Here's how the part is built. I have some questions about the finished solid (model axes, mm). Coordinates: 2 decimals unless noted, no trailing zeros. Write each loop counter-clockwise with the first axis right and the second up, starting at its lowest first coordinate (ties: lowest second). Pieces come first, ordered by that corner, then holes.
Autodesk Inventor part; units mm, degrees
ref_plane "YZ Plane" through (0, 0, 0) normal (1, 0, 0) x (0, 1, 0)
ref_plane "XZ Plane" through (0, 0, 0) normal (0, 1, 0) x (-1, 0, 0)
ref_plane "XY Plane" through (0, 0, 0) normal (0, 0, 1) x (1, 0, 0)
sketch "Sketch1" plane through (0, 0, 0) normal (0, 1, 0) x (-1, 0, 0)
  line L0 (0, 0) -> (1000, 0)
  line L1 (1000, 0) -> (1000, 1500)
  line L2 (1000, 1500) -> (0, 1500)
  line L3 (0, 1500) -> (0, 0)
  dimension "d0" = 1000
  dimension "d1" = 1500
extrude "base" add sketch "Sketch1" along normal blind 150
sketch "Sketch2" plane through (0, 150, 0) normal (0, 1, 0) x (1, 0, 0)
  circle A0 centre (-500, -700) radius 57.5
  line L0 (0, 0) -> (-1000, 0)
  line L1 (-1000, -1500) -> (0, -1500)
  line L2 (-500, 0) -> (-500, -1500) construction
  dimension "d4" = 115
  dimension "d38" = 700
extrude "air" cut sketch "Sketch2" against normal through all
sketch "Sketch3" plane through (0, 150, 0) normal (0, 1, 0) x (1, 0, 0)
  circle A0 centre (-500, -700) radius 57.5
  circle A1 centre (-400, -200) radius 24.5
  circle A2 centre (-600, -200) radius 24.5
  line L0 (0, 0) -> (-1000, 0)
  dimension "d7" = 49
  dimension "d40" = 100
  dimension "d41" = 49
  dimension "d42" = 100
  dimension "d55" = 200
extrude "power" cut sketch "Sketch3" against normal blind 254 contours A1 | A2
sketch "Sketch4" plane through (0, 150, 0) normal (0, 1, 0) x (1, 0, 0)
  circle A0 centre (-600, -200) radius 24.5
  circle A1 centre (-500, -500) radius 24.5
  line L0 (0, 0) -> (-1000, 0)
  dimension "d52" = 49
  dimension "d53" = 500
hole "fibre" at (-500, 150, 500) direction (0, -1, 0) diameter 45 end through all
sketch "Sketch6" plane through (0, 150, 0) normal (0, 1, 0) x (1, 0, 0)
  circle A0 centre (-500, -700) radius 57.5
  circle A1 centre (-500, -1350) radius 76.2
  dimension "d29" = 152.4
  dimension "d30" = 650
hole "air2" at (-500, 150, 1350) direction (0, -1, 0) diameter 115 end through all
properties part number "plinth" material "Concrete"
1) Imagine slicing it at D-D on z = 200. Please give me the cut outline in (x, y).
Values follow:
outline: (-1000, 0) - (-624.5, 0) - (-624.5, 150) - (-1000, 150) - close; (-575.5, 0) - (-424.5, 0) - (-424.5, 150) - (-575.5, 150) - close; (-375.5, 0) - (0, 0) - (0, 150) - (-375.5, 150) - close
2) Imagine slicing it at C-C on x = -500. Please give me the cut outline in (y, z), then the cut area to 3 significant figures.
Values follow:
outline: (0, 0) - (150, 0) - (150, 477.5) - (0, 477.5) - close; (0, 522.5) - (150, 522.5) - (150, 642.5) - (0, 642.5) - close; (0, 757.5) - (150, 757.5) - (150, 1292.5) - (0, 1292.5) - close; (0, 1407.5) - (150, 1407.5) - (150, 1500) - (0, 1500) - close
area: 184,000 mm2
3) Imagine slicing it at A-A on x = -600. Please give me the cut outline in (y, z).
Values follow:
outline: (0, 0) - (150, 0) - (150, 175.5) - (0, 175.5) - close; (0, 224.5) - (150, 224.5) - (150, 1500) - (0, 1500) - close
4) Imagine slicing it at B-B on z = 500. Please give me the cut outline in (x, y), then the cut area to 3 significant figures.
Values follow:
outline: (-1000, 0) - (-522.5, 0) - (-522.5, 150) - (-1000, 150) - close; (-477.5, 0) - (0, 0) - (0, 150) - (-477.5, 150) - close
area: 143,000 mm2
5) I need wall thicknesses on probe 1 along Z at (x, y) = (-500, 34); probe 2 along Z at (x, y) = (-508.5, 80); probe 3 along X at (y, z) = (117, 219.5). Which ranges of each line are inside material? Lowest first, please.
Values follow:
probe 1: z = 0 to 477.5, 522.5 to 642.5, 757.5 to 1292.5, 1407.5 to 1500
probe 2: z = 0 to 479.17, 520.83 to 643.13, 756.87 to 1293.13, 1406.87 to 1500
probe 3: x = -1000 to -614.83, -585.17 to -414.83, -385.17 to 0
6) We'd pull the mould along X, two halves only. Please class faces 1 (the face through (-493, 150, 760)), 2 (the face through (-618.058, 76.05, 183.442)), 3 (the face through (-506.76, 73.95, 521.46)), 4 (the face through (0, 74, 760)): pulls with the +X half, pulls with the -X half, needs draft (parallel to the pull), parting line crosses it, or undercut.
Values follow:
face 1: needs draft
face 2: undercut
face 3: undercut
face 4: pulls with the +X half
